Source: CAD feature listing. Evaluate the final solid. Frame: model axes, mm. A direction names the side the tool comes from. Round coordinates to 2 decimals unless told otherwise and drop trailing zeros. Loops run counter-clockwise (first coordinate to the right, second up) from the corner with the lowest first, then second, coordinate; pieces in that order, holes last.
(1) Material intervals for probe 1 along X at (y, z) = (63, 10.5) (3 decimals); probe 2 along Z at (x, y) = (114, 5) (3 decimals); probe 3 along Z at (x, y) = (7, 27) (3 decimals), sorted ascending.
(2) Mould query, pull axis Z, two halves, no side actions, for faces 6 (the flat face through (-70.85, 30.78, 59)), 7 (the flat face through (0, 16, 68.58)), 8 (the flat face through (13.168, 47, 54)). Classes: pulls with the +Z half, pulls with the -Z half, needs draft (parallel to the pull), parting line crosses it, or undercut.
(3) Section A-A, the plane x = 59. Return the cut outline in (y, z) (3 decimals).
(4) First-contact query: pin 1 Ø2 at (x, z) = (-34.5, 10) entering from -Y (3 decimals); pin 2 Ø14 at (x, y) = (-79, 4) entering from +Z; pin 3 Ø13 at (x, y) = (-86, 4) entering from -Z; pin 4 Ø19.5 at (x, z) = (-53, 23) entering from -Y. Flat tips, straight axial feed; report the tip coordinate or a pass-through.
(5) Section D-D, the plane y = 46. Return the cut outline in (x, z) (3 decimals), plus the area to 3 significant figures.
(6) Set-up query: faces 1 (the flat face through (-127, 29, 28)), 2 (the flat face through (-13.168, 47, 54)), 3 (the flat face through (72.49, 30.78, 59)), 4 (the flat face through (-0.184, 54.286, 57.598)), 5 (the flat face through (0, 16, 71.12)). Return all of +Z, -Z, +X, -X, +Y, -Y with unobstructed straight access to the full face (end or side cutting, diameter ignored); none if empty.
(7) Section B-B, the plane z = 25. Return the cut outline in (x, y) (3 decimals).
(8) Section C-C, the plane y = 9.5. Return the cut outline in (x, z) (3 decimals), plus the area to 3 significant figures.
```python
from build123d import *

# Parameters (mm, degrees)
BOSS_EXTRUDE1_DEPTH = 127
BOSS_EXTRUDE2_DEPTH = 3.175
SKETCH3_W           = 63.5
SKETCH3_H           = 30.48
CUT_EXTRUDE1_DEPTH  = 3.175
BOSS_EXTRUDE3_START = -13.167941481
BOSS_EXTRUDE3_DEPTH = 26.335882962
SKETCH10_W          = 26.335882962
SKETCH10_H          = 12.7
BOSS_EXTRUDE5_DEPTH = 31.75
CUT_EXTRUDE7_START  = -10.627941481
CUT_EXTRUDE7_DEPTH  = 21.255882962
CUT_EXTRUDE8_START  = -2.54
SKETCH12_W          = 21.255882962
SKETCH12_H          = 31.75
CUT_EXTRUDE8_DEPTH  = 15.24
CUT_EXTRUDE9_START  = -26.335883
CUT_EXTRUDE9_DEPTH  = 26.335883


# Read off the part's stored shape, not the designer's step: Boss-Extrude3, Cut-Extrude7
with BuildPart() as part:
    # Sketch1 → Boss-Extrude1 (new, symmetric)
    with BuildSketch(Plane(origin=(0, 0, 0), x_dir=(0, 0, -1), z_dir=(1, 0, 0))):
        Polygon((-3.175, 0), (0, 0), (0, 76.2), (-31.75, 76.2), (-69.85, 12.7), (-69.85, 0), (-66.675, 0), (-66.675, 11.820575911), (-29.952345547, 73.025), (-3.175, 73.025), align=None)
    extrude(amount=BOSS_EXTRUDE1_DEPTH, both=True)

    # Sketch2 → Boss-Extrude2 (add)
    with BuildSketch(Plane(origin=(127, 0, 0), x_dir=(0, 0, -1), z_dir=(1, 0, 0))):
        Polygon((-66.675, 0), (-3.175, 0), (-3.175, 73.025), (-29.952345547, 73.025), (-66.675, 11.820575911), align=None)
        Polygon((-66.675, 11.820575911), (-29.952345547, 73.025), (-3.175, 73.025), (-3.175, 0), (0, 0), (0, 76.2), (-31.75, 76.2), (-69.85, 12.7), (-69.85, 0), (-66.675, 0), align=None)
    boss_extrude2 = extrude(amount=BOSS_EXTRUDE2_DEPTH)

    # Mirror1: Boss-Extrude2 across plane
    add(boss_extrude2.mirror(Plane(origin=(0, 0, 0), x_dir=(0, 0, 1), z_dir=(1, 0, 0))))

    # Sketch3 → Cut-Extrude1 (cut)
    with BuildSketch(Plane(origin=(0, 34.177941176, 56.963235294), x_dir=(1, 0, 0), z_dir=(0, 0.5144957554275267, 0.8574929257125442))):
        with Locations((-67.993455951, 13.879941606)):
            Rectangle(SKETCH3_W, SKETCH3_H)
        with Locations((67.993455951, 13.879941606)):
            Rectangle(SKETCH3_W, SKETCH3_H)
    extrude(amount=-CUT_EXTRUDE1_DEPTH, mode=Mode.SUBTRACT)

    # Boss-Extrude3 outline → Boss-Extrude3 (add)
    with BuildSketch(Plane.YZ.offset(BOSS_EXTRUDE3_START)):
        Polygon((76.2, 31.75), (76.2, 44.45), (31.75, 71.12), (31.75, 58.42), align=None)
    extrude(amount=BOSS_EXTRUDE3_DEPTH)

    # Sketch10 → Boss-Extrude5 (add)
    with BuildSketch(Plane.XZ.offset(-31.75)):
        with Locations((0, 64.77)):
            Rectangle(SKETCH10_W, SKETCH10_H)
    extrude(amount=BOSS_EXTRUDE5_DEPTH)

    # Cut-Extrude7 outline → Cut-Extrude7 (cut)
    with BuildSketch(Plane.YZ.offset(CUT_EXTRUDE7_START)):
        Polygon((31.75, 54.717345547), (73.025, 29.952345547), (73.025, 42.652345547), (31.75, 67.417345547), align=None)
    extrude(amount=CUT_EXTRUDE7_DEPTH, mode=Mode.SUBTRACT)

    # Sketch12 → Cut-Extrude8 (cut)
    with BuildSketch(Plane.XY.offset(71.12).offset(CUT_EXTRUDE8_START)):
        with Locations((0, 15.875)):
            Rectangle(SKETCH12_W, SKETCH12_H)
    extrude(amount=-CUT_EXTRUDE8_DEPTH, mode=Mode.SUBTRACT)

    # Sketch13 → Cut-Extrude9 (cut)
    with BuildSketch(Plane(origin=(13.167941481, 0, 0), x_dir=(0, 0, -1), z_dir=(1, 0, 0)).offset(CUT_EXTRUDE9_START)):
        Polygon((-58.42, 25.578909245), (-66.675, 11.820575911), (-66.675, 0), (-58.42, 0), align=None)
    extrude(amount=CUT_EXTRUDE9_DEPTH, mode=Mode.SUBTRACT)


solid = part.part
```
Output values:
1. probe 1: x = -130.175 to -127, 127 to 130.175
1. probe 2: z = 0 to 3.175, 66.675 to 69.85
1. probe 3: z = 0 to 3.175, 68.58 to 71.12
2. face 6: pulls with the +Z half
2. face 7: undercut
2. face 8: needs draft
3. outline: (0, 0) - (76.2, 0) - (76.2, 31.75) - (59.148, 41.981) - (57.515, 39.259) - (73.025, 29.952) - (73.025, 3.175) - (0, 3.175) - close; (0, 66.675) - (11.821, 66.675) - (31.378, 54.94) - (33.012, 57.663) - (12.7, 69.85) - (0, 69.85) - close
4. pin 1: stops at y = 73.025
4. pin 2: stops at z = 69.85
4. pin 3: stops at z = 0
4. pin 4: stops at y = 68.36
5. outline: (-130.175, 0) - (130.175, 0) - (130.175, 49.87) - (99.743, 49.87) - (99.743, 46.167) - (127, 46.167) - (127, 3.175) - (-127, 3.175) - (-127, 46.167) - (-99.743, 46.167) - (-99.743, 49.87) - (-130.175, 49.87) - close; (-36.243, 46.167) - (-10.628, 46.167) - (-10.628, 58.867) - (10.628, 58.867) - (10.628, 46.167) - (36.243, 46.167) - (36.243, 49.87) - (13.168, 49.87) - (13.168, 62.57) - (-13.168, 62.57) - (-13.168, 49.87) - (-36.243, 49.87) - close
5. area: 1,660 mm2
6. face 1: -Y
6. face 2: +Z, -X, +Y
6. face 3: +Z, +X, +Y
6. face 4: +Z, +X, -X, +Y
6. face 5: +Z, +X, -X, +Y, -Y
7. outline: (-130.175, 0) - (-127, 0) - (-127, 73.025) - (127, 73.025) - (127, 0) - (130.175, 0) - (130.175, 76.2) - (-130.175, 76.2) - close
8. outline: (-130.175, 0) - (130.175, 0) - (130.175, 69.85) - (13.168, 69.85) - (13.168, 71.12) - (-13.168, 71.12) - (-13.168, 69.85) - (-130.175, 69.85) - close; hole (-127, 3.175) - (127, 3.175) - (127, 66.675) - (10.628, 66.675) - (10.628, 68.58) - (-10.628, 68.58) - (-10.628, 66.675) - (-127, 66.675) - close
8. area: 2,050 mm2
